from build123d import *

# Parameters (mm, degrees)
SKETCH_1_W          = 164.5
SKETCH_1_H          = 100
EXTRUDE_1_DEPTH     = 25
SKETCH_2_W          = 103
SKETCH_2_H          = 100
EXTRUDE_2_DEPTH     = 65
SKETCH_5_R          = 31.5
CUT_EXTRUDE_3_DEPTH = 125
CUT_EXTRUDE_4_DEPTH = 1


with BuildPart() as part:
    # Sketch 1 → Extrude 1 (new body)
    with BuildSketch(Plane(origin=(0, 0, 0), x_dir=(1, 0, 0), z_dir=(0, 1, 0))):
        with Locations((82.25, 50)):
            Rectangle(SKETCH_1_W, SKETCH_1_H)
    extrude(amount=EXTRUDE_1_DEPTH)

    # Sketch 2 → Extrude 2 (add)
    with BuildSketch(Plane(origin=(0, 25, 0), x_dir=(1, 0, 0), z_dir=(0, 1, 0))):
        with Locations((51.5, 50)):
            Rectangle(SKETCH_2_W, SKETCH_2_H)
    extrude(amount=EXTRUDE_2_DEPTH)

    # Sketch 5 → Cut-Extrude 3 (cut)
    with BuildSketch(Plane(origin=(0, 90, 0), x_dir=(1, 0, 0), z_dir=(0, 1, 0))):
        with Locations(Location((46.5, 50, 0), (0, 0, 270))):
            Circle(SKETCH_5_R)
    extrude(amount=-CUT_EXTRUDE_3_DEPTH, mode=Mode.SUBTRACT)

    # Sketch 6 → Cut-Extrude 4 (cut)
    with BuildSketch(Plane(origin=(0, 90, 0), x_dir=(1, 0, 0), z_dir=(0, 1, 0))):
        with BuildLine():
            Line((81.59399548, 80.506744848), (81.59399548, 19.493255152))
            ThreePointArc((81.59399548, 19.493255152), (46.5, 3.5), (11.40600452, 19.493255152))
            Line((11.40600452, 19.493255152), (11.40600452, 80.506744848))
            ThreePointArc((11.40600452, 80.506744848), (46.5, 96.5), (81.59399548, 80.506744848))
        make_face()
    extrude(amount=-CUT_EXTRUDE_4_DEPTH, mode=Mode.SUBTRACT)


solid = part.part
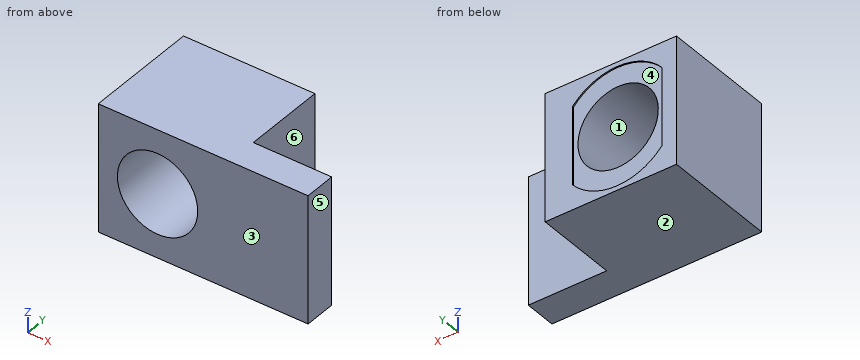
Work out the finished part from the listing and answer in its coordinate system (mm). Face numbers are marked on the shaded views. A direction names the side the tool comes from. Round coordinates to 2 decimals unless told otherwise and drop trailing zeros. Write each loop counter-clockwise with the first axis right and the second up, starting at its lowest first coordinate (ties: lowest second). Pieces come first, ordered by that corner, then holes. Notation, with made-up numbers: (81, 80) -> (103, 80) arc R21 ccw to (103, 94) -> close; hole circle Ø6 at (71, 6). An arc over 180 degrees is marked (long way). Answer as CSV lines item,"result". Start each with the question number.
(1) Each of these flat-tipped pins is pushed along its axis until it touches: pin 1 (6 mm diameter, centred on x = 24, y = 41.5, fed in from +Z); pin 2 (4 mm diameter, centred on y = 30, z = -74, fed in from +X); pin 3 (21 mm diameter, centred on x = 63.5, z = -69, fed in from +Y). Where does it stop, or does it pass through?
(2) The part is cut by section B-B, the plane x = 46.5. Give the vertices of the cut face in (y, z), then the cut area to 3 significant figures.
(3) The part is cut by section A-A, the plane z = -50. Give the vertices of the cut face in (x, y), then the cut area to 3 significant figures.
(4) The part is cut by section D-D, the plane z = -31.5. Give the vertices of the cut face in (x, y).
(5) The part is cut by section C-C, the plane y = 61. Give the vertices of the cut face in (x, z), then the cut area to 3 significant figures.
(6) Find the intervals of material crossed by probe 1 along X at (y, z) = (42.5, -49); probe 2 along Z at (x, y) = (46, 54); probe 3 along Y at (x, z) = (34, -81), in increasing order.
(7) A tool of negligible diameter and unlimited length cuts with its end or side. For the marked faces 4, 5 and 6, from which of +Z, -Z, +X, -X, +Y, -Y can it reach the whole face along a straight path? Write none if from no direction.
(8) The mould has two halves that part along Z. Classify the marked faces 1, 2 and 3: +Z half, -Z half, draft (parallel to the pull), parting line (faces both ways), or undercut.
Output values:
1,pin 1,"stops at z = 0"
1,pin 2,"stops at x = 103"
1,pin 3,"stops at y = 89"
2,outline,"(0, -100) -> (90, -100) -> (90, -96.5) -> (89, -96.5) -> (89, -81.5) -> (0, -81.5) -> close; (0, -18.5) -> (89, -18.5) -> (89, -3.5) -> (90, -3.5) -> (90, 0) -> (0, 0) -> close"
2,area,"3,300 mm²"
3,outline,"(0, 0) -> (15, 0) -> (15, 89) -> (11.41, 89) -> (11.41, 90) -> (0, 90) -> close; (78, 0) -> (164.5, 0) -> (164.5, 25) -> (103, 25) -> (103, 90) -> (81.59, 90) -> (81.59, 89) -> (78, 89) -> close"
3,area,"5,130 mm²"
4,outline,"(0, 0) -> (21, 0) -> (21, 89) -> (11.41, 89) -> (11.41, 90) -> (0, 90) -> close; (72, 0) -> (164.5, 0) -> (164.5, 25) -> (103, 25) -> (103, 90) -> (81.59, 90) -> (81.59, 89) -> (72, 89) -> close"
5,outline,"(0, -100) -> (103, -100) -> (103, 0) -> (0, 0) -> close; hole circle Ø63 at (46.5, -50)"
5,area,"7,180 mm²"
6,probe 1,"x = 0 to 15.02, 77.98 to 103"
6,probe 2,"z = -100 to -81.5, -18.5 to 0"
6,probe 3,"y = 0 to 89"
7,face 4,"+Y"
7,face 5,"+Z, -Z, +X, +Y, -Y"
7,face 6,"+Z, -Z, +X, +Y"
8,face 1,"undercut"
8,face 2,"-Z half"
8,face 3,"draft"
